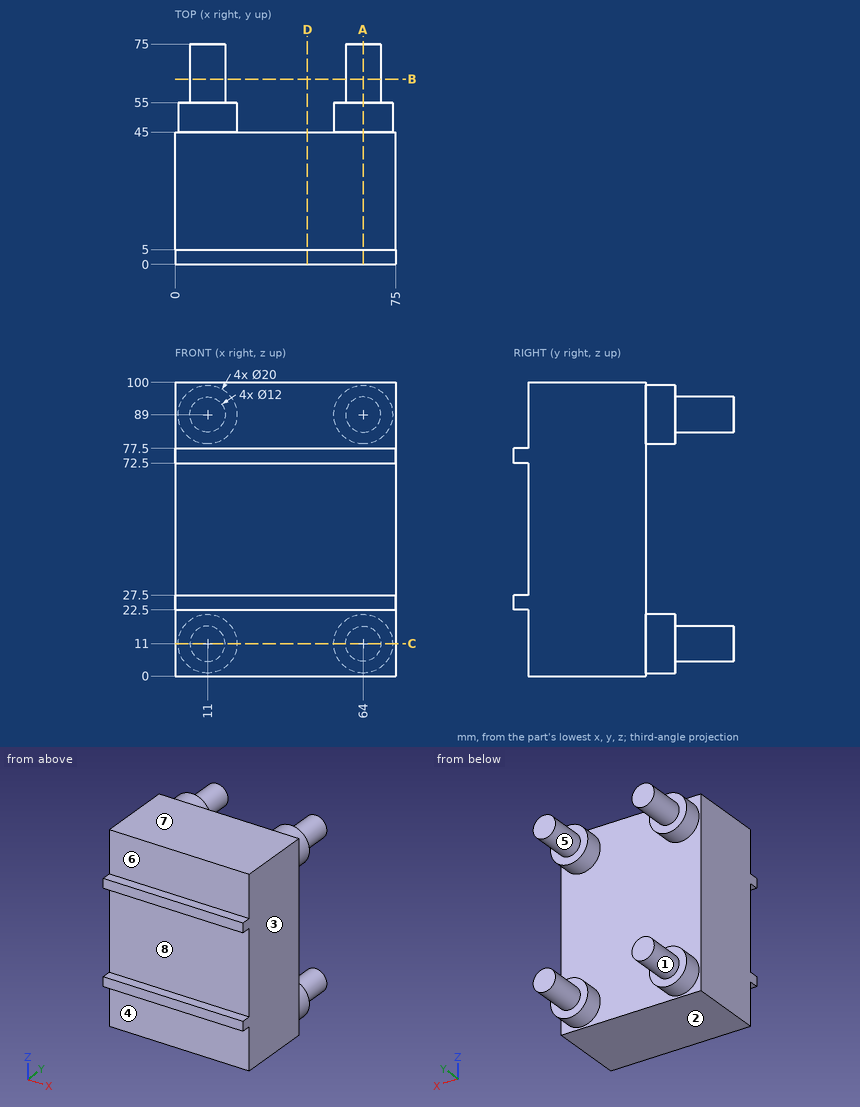
Drawing for the job (mm, zero at the part's lowest x, y, z). A direction names the side the tool comes from. Round coordinates to 2 decimals unless told otherwise and drop trailing zeros. Write each loop counter-clockwise with the first axis right and the second up, starting at its lowest first coordinate (ties: lowest second). Pieces come first, ordered by that corner, then holes. Notation, with made-up numbers: M 83.25,6 L 90.25,6 A30 ccw 90.25,37 Z; hole C -24.75,79.25 d11. An arc over 180 degrees is marked long. Answer as a JSON object with one key per item and string values. Group by question number.
(1) Which spindle directions (+Z, -Z, +X, -X, +Y, -Y) get a long thin tool onto all of the face, cutting with end or side? Do the marked faces 4, 5, 6, 7 and 8. Say none if no direction does.
(2) Mould opens along X. For the marked faces 1, 2 and 3 say: pulls with the +X half, pulls with the -X half, needs draft (parallel to the pull), parting line crosses it, or undercut.
(3) Cut at A-A (x = 64). Give the cut face in (y, z).
(4) Cut at D-D (x = 45). Give the cut face in (y, z), and give its area (3 significant figures).
(5) Flat gauge pins, fed straight in: pin 1 (13.5 mm diameter, centred on x = 47, z = 40, fed in from -Y); pin 2 (5.5 mm diameter, centred on x = 48.5, y = 2.5, fed in from -Z); pin 3 (12 mm diameter, centred on y = 52.5, z = 45.5, fed in from -X) (3 decimals); pin 4 (2.5 mm diameter, centred on x = 28, y = 2, fed in from +Z). Where does each tip first touch, or does it go through?
(6) Cut at B-B (y = 63). Give the cut face in (x, z), and give its area (3 significant figures).
(7) Cut at C-C (z = 11). Give the cut face in (x, y).
(8) Drill centre lines: L1, parallel to Y at x = 21, z = 73; L2, parallel to Z at x = 62, y = 68.5; L3, parallel to Y at x = 70, z = 54.5. Where is each one in solid material? Low to high.
Responses:
{
 "1": {"face 4": "-Z, +X, -X, -Y", "face 5": "+Y", "face 6": "+Z, +X, -X, -Y", "face 7": "+Z, +X, -X, +Y, -Y", "face 8": "+X, -X, -Y"},
 "2": {"face 1": "undercut", "face 2": "needs draft", "face 3": "pulls with the +X half"},
 "3": {"outline": "M 0,22.5 L 5,22.5 L 5,0 L 45,0 L 45,1 L 55,1 L 55,5 L 75,5 L 75,17 L 55,17 L 55,21 L 45,21 L 45,79 L 55,79 L 55,83 L 75,83 L 75,95 L 55,95 L 55,99 L 45,99 L 45,100 L 5,100 L 5,77.5 L 0,77.5 L 0,72.5 L 5,72.5 L 5,27.5 L 0,27.5 Z"},
 "4": {"outline": "M 0,22.5 L 5,22.5 L 5,0 L 45,0 L 45,100 L 5,100 L 5,77.5 L 0,77.5 L 0,72.5 L 5,72.5 L 5,27.5 L 0,27.5 Z", "area": "4,050 mm2"},
 "5": {"pin 1": "stops at y = 5", "pin 2": "stops at z = 0", "pin 3": "passes through", "pin 4": "stops at z = 77.5"},
 "6": {"outline": "C 11,11 d12; C 11,89 d12; C 64,11 d12; C 64,89 d12", "area": "452 mm2"},
 "7": {"outline": "M 0,5 L 75,5 L 75,45 L 74,45 L 74,55 L 70,55 L 70,75 L 58,75 L 58,55 L 54,55 L 54,45 L 21,45 L 21,55 L 17,55 L 17,75 L 5,75 L 5,55 L 1,55 L 1,45 L 0,45 Z"},
 "8": {"L1": "y = 0 to 45", "L2": "z = 5.34 to 16.66, 83.34 to 94.66", "L3": "y = 5 to 45"}
}
